```python
from build123d import *

# Parameters (mm, degrees)
SKETCH_W               = 200
SKETCH_H               = 110
PAD_DEPTH              = 10
HOLE_D                 = 8.8
HOLE_CSINK_D           = 16
HOLE_CSINK_ANGLE       = 90
LINEARPATTERN_COUNT    = 2
LINEARPATTERN_PITCH    = 40
SKETCH002_R            = 3.3
HOLE001_DEPTH          = 10.001
LINEARPATTERN001_COUNT = 2
LINEARPATTERN001_PITCH = 55
HOLE002_D              = 8.8
HOLE002_CSINK_D        = 16
HOLE002_CSINK_ANGLE    = 90
LINEARPATTERN002_COUNT = 4
LINEARPATTERN002_PITCH = 40


with BuildPart() as part:
    # Sketch → Pad (new body)
    with BuildSketch(Plane.XY):
        with Locations((100, 55)):
            Rectangle(SKETCH_W, SKETCH_H)
    extrude(amount=PAD_DEPTH)

    # Hole (through all)
    with Locations(Plane.XY.offset(10)):
        with Locations((20, 20)):
            hole = CounterSinkHole(HOLE_D / 2, HOLE_CSINK_D / 2, counter_sink_angle=HOLE_CSINK_ANGLE)

    # LinearPattern: Hole ×2
    with Locations(*[(0, i * LINEARPATTERN_PITCH, 0) for i in range(1, LINEARPATTERN_COUNT)]):
        add(hole, mode=Mode.SUBTRACT)

    # Sketch002 → Hole001 (cut, through all)
    with BuildSketch(Plane.XY.offset(10)):
        with Locations((180, 63)):
            Circle(SKETCH002_R)
    hole001 = extrude(amount=-HOLE001_DEPTH, mode=Mode.SUBTRACT)

    # LinearPattern001: Hole001 ×2
    with Locations(*[(0, -i * LINEARPATTERN001_PITCH, 0) for i in range(1, LINEARPATTERN001_COUNT)]):
        add(hole001, mode=Mode.SUBTRACT)

    # Hole002 (through all)
    with Locations(Plane.XY.offset(10)):
        with Locations((40, 90)):
            hole002 = CounterSinkHole(HOLE002_D / 2, HOLE002_CSINK_D / 2, counter_sink_angle=HOLE002_CSINK_ANGLE)

    # LinearPattern002: Hole002 ×4
    with Locations(*[(i * LINEARPATTERN002_PITCH, 0, 0) for i in range(1, LINEARPATTERN002_COUNT)]):
        add(hole002, mode=Mode.SUBTRACT)


solid = part.part
```
Check sheet for the modelled part. Datum: model origin and axes. Units: mm. Give positions to 0.01 mm unless a question says otherwise; leave off trailing zeros. Loops run counter-clockwise (first coordinate to the right, second up) from the corner with the lowest first, then second, coordinate; pieces in that order, holes last. Notation, with made-up numbers: M -6.5,8.25 L 30.5,8.25 A21 cw 30.5,35.25 Z; hole C -16,89.5 d3. An arc over 180 degrees is marked long. Answer in a Markdown table with one row per item.
1) Depth check by flat-ended pin: pin 1 (10 mm diameter, centred on x = 160, y = 90, fed in from +Z). Enter the tip coordinate at first touch or a pass-through.
Solutions:
| item | result |
|---|---|
| pin 1 | stops at z = 7 |
2) Thickness scan on line 1 (X direction, y = 90, z = 3.5); line 2 (Y direction, x = 160, z = 3.5); line 3 (X direction, y = 60, z = 3). Record the ranges inside material, lowest first.
Solutions:
| item | result |
|---|---|
| line 1 | x = 0 to 35.6, 44.4 to 75.6, 84.4 to 115.6, 124.4 to 155.6, 164.4 to 200 |
| line 2 | y = 0 to 85.6, 94.4 to 110 |
| line 3 | x = 0 to 15.6, 24.4 to 178.63, 181.37 to 200 |
3) Mould release check, pull along X, two halves, no side actions. Record for faces 1 (the face through (15.64, 21.37, 6.57)), 2 (the face through (99, 110, 5)), 3 (the face through (0, 54, 5)): released by +X, released by -X, zero draft, split by the parting line, or undercut.
Solutions:
| item | result |
|---|---|
| face 1 | undercut |
| face 2 | zero draft |
| face 3 | released by -X |
4) Cross-section at D-D (y = 8). Enter the section's corners in (x, z).
Solutions:
| item | result |
|---|---|
| outline | M 0,0 L 176.7,0 L 176.7,10 L 0,10 Z; M 183.3,0 L 200,0 L 200,10 L 183.3,10 Z |
5) Cross-section at C-C (x = 180). Enter the section's corners in (y, z).
Solutions:
| item | result |
|---|---|
| outline | M 0,0 L 4.7,0 L 4.7,10 L 0,10 Z; M 11.3,0 L 59.7,0 L 59.7,10 L 11.3,10 Z; M 66.3,0 L 110,0 L 110,10 L 66.3,10 Z |
6) Cross-section at A-A (x = 120). Enter the section's corners in (y, z), plus the area to 3 significant figures.
Solutions:
| item | result |
|---|---|
| outline | M 0,0 L 85.6,0 L 85.6,6.4 L 82,10 L 0,10 Z; M 94.4,0 L 110,0 L 110,10 L 98,10 L 94.4,6.4 Z |
| area | 999 mm^2 |
7) Cross-section at B-B (z = 1.5). Count the separate pieces of the cut face and the enclosed holes in it, plus the area to 3 significant figures.
Solutions:
| item | result |
|---|---|
| separate pieces | 1 |
| enclosed holes | 8 |
| area | 21,600 mm^2 |
